Read the model definition and answer for the solid it produces. Units are mm, in the model's axes. Face numbers are marked on the shaded views. A direction names the side the tool comes from. Coordinates: 2 decimals unless noted, no trailing zeros. Order: outer loops, then holes, each group sorted by start corner. A loop starts at its lowest first (then second) coordinate and runs counter-clockwise, first axis right, second up.
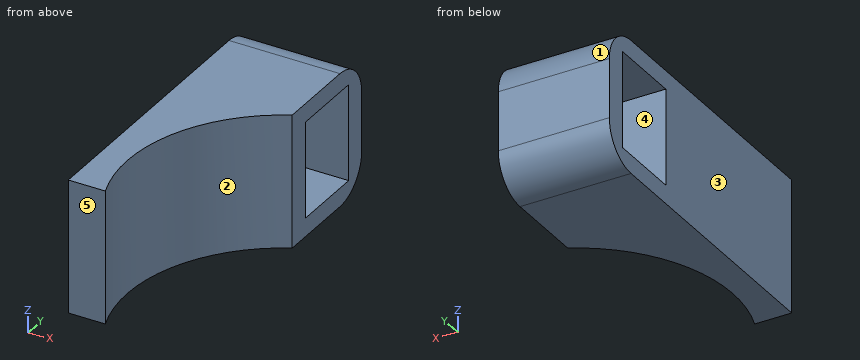
from build123d import *

# Parameters (mm, degrees)
F0_W     = 15
F0_H     = 12
F1_DEPTH = 18
F2_W     = 10
F2_H     = 13
F3_DEPTH = 25
F4_R     = 5


with BuildPart() as f1:
    # F0 (on Top) → F1 (new body)
    with BuildSketch(Plane.XY):
        with BuildLine():
            Line((0, 30), (0, 0))
            Line((0, 0), (5, 0))
            ThreePointArc((5, 0), (5.06842, 14.896762), (15, 26))
            Line((15, 26), (15, 30))
            Line((15, 30), (0, 30))
        make_face()
        with Locations((7.5, 36)):
            Rectangle(F0_W, F0_H)
    extrude(amount=F1_DEPTH)

    # F2 (on face) → F3 (cut)
    with BuildSketch(Plane.YZ.offset(15)):
        with Locations((34, 9)):
            Rectangle(F2_W, F2_H)
    extrude(amount=-F3_DEPTH, mode=Mode.SUBTRACT)

    # F4
    f4_edges = [f1.edges().sort_by_distance(p)[0] for p in [
        (7.5, 42, 18),
        (7.5, 42, 0),
    ]]
    fillet(f4_edges, radius=F4_R)


solid = f1.part
Q1. The part is cut by section C-C, the plane y = 35. Determine the outline of the cut face in (x, z).
Q2. Determine the mould class of the marked faces 1, 2 and 3 for opening direction Y: +Y half, -Y half, draft (parallel to the pull), parting line (faces both ways), or undercut.
Q3. Which of the six approach directions +Z, -Z, +X, -X, +Y, -Y give full straight-line access (tool end or side, diameter ignored) to the marked faces 4 and 5?
Q4. The part is cut by section A-A, the plane z = 6.5. Determine the outline of the cut face in (x, y), then the cut area to 3 significant figures.
Q5. The part is cut by section D-D, the plane z = 4. Determine the outline of the cut face in (x, y).
Q6. Straight lines are drawn through the part: L1, parallel to Z at x = 14.25, y = 31; L2, parallel to X at y = 7, z = 9.75; L3, parallel to Y at x = 8.5, z = 12.75. For each, find the intervals that lie inside material, in ascending order.
Q7. Each of these flat-tipped pins is pushed along its axis until it touches: P1, Ø1, axis at y = 15.5, z = 8.5, coming from the -X side; P2, Ø4, axis at x = 9.5, z = 10, coming from the -Y side; P3, Ø1.5, axis at x = 8, z = 13, coming from the -Y side. Where does it stop, or does it pass through?
Q8. The part is cut by section B-B, the plane x = 2. Determine the outline of the cut face in (y, z).
Computed values:
1. outline: (0, 0) - (15, 0) - (15, 2.5) - (0, 2.5) - close; (0, 15.5) - (15, 15.5) - (15, 18) - (0, 18) - close
2. face 1: +Y half
2. face 2: undercut
2. face 3: draft
3. face 4: +X, -X
3. face 5: +Z, -Z, +X, -X, -Y
4. outline: (0, 0) - (5, 0) arc R21 cw to (15, 26) - (15, 29) - (0, 29) - close; (0, 39) - (15, 39) - (15, 42) - (0, 42) - close
4. area: 249 mm2
5. outline: (0, 0) - (5, 0) arc R21 cw to (15, 26) - (15, 29) - (0, 29) - close; (0, 39) - (15, 39) - (15, 41.9) - (0, 41.9) - close
6. L1: z = 0 to 2.5, 15.5 to 18
6. L2: x = 0 to 3.67
6. L3: y = 20.76 to 29, 39 to 42
7. P1: stops at x = 0
7. P2: stops at y = 19.45
7. P3: stops at y = 19.09
8. outline: (0, 0) - (37, 0) arc R5 ccw to (42, 5) - (42, 13) arc R5 ccw to (37, 18) - (0, 18) - close; hole (29, 2.5) - (39, 2.5) - (39, 15.5) - (29, 15.5) - close
